Design review of the part built by this model. Coordinates are the model's own, in mm. A direction names the side the tool comes from. Round coordinates to 2 decimals unless told otherwise and drop trailing zeros. Write each loop counter-clockwise with the first axis right and the second up, starting at its lowest first coordinate (ties: lowest second). Pieces come first, ordered by that corner, then holes. Notation, with made-up numbers: (81, -5) -> (101, -5) arc R24 cw to (101, 26) -> close; hole circle Ø1 at (52, -14). An arc over 180 degrees is marked (long way). Write item = value, one per line. Start each with the question number.
Item 1: Add section D-D, the plane x = 132. State the section outline as (y, z) points.
Item 2: Add section C-C, the plane z = 96. State the section outline as (x, y) points, then the cut area to 3 significant figures.
Item 3: Add section B-B, the plane x = 15. State the section outline as (y, z) points (3 decimals).
Item 4: Add section A-A, the plane y = -4.25. State how many separate pieces and enclosed holes the cut face has, then the cut area to 3 significant figures.
Item 5: To check wall thickness, follow L1, parallel to X at y = -1.5, z = -26.5 (3 decimals); L2, parallel to X at y = -2.5, z = 23 (3 decimals); L3, parallel to Z at x = 15, y = -5.1 (3 decimals). State the ranges of each line that lie inside material, in increasing order.
Item 6: For pin 1 Ø10 at (x, z) = (-15, 25.98) entering from +Y; pin 2 Ø4 at (x, z) = (15, -25.98) entering from +Y; pin 3 Ø8.5 at (x, z) = (-30, 0) entering from +Y, all flat-tipped, find the tip position at first contact; note any pin that passes through.
Item 7: Mouldability with a two-part tool opening along X and no side actions: class faces 3 (the flat face through (-60, -3, 169.625)), 4 (the conical face through (-18.27, -2.95, 26.71)), 5 (the cylindrical face through (-71.484, -3.131, -69.929)) as released by +X, released by -X, zero draft, split by the parting line, or undercut.
Item 8: Machinability: for faces 1 (the flat face through (-20, -3, 123)), 2 (the conical face through (33.32, -2.95, 0.44)), which of the approach directions +Z, -Z, +X, -X, +Y, -Y give a long, thin tool a straight path to every point of the face, cutting with its end or side? Answer none if there is none.
from build123d import *

# Parameters (mm, degrees)
BOSS_EXTRUDE1_DEPTH                             = 6.35
FILLET1_R                                       = 5
TAP_DRILL_FOR_M6X1_0_TAP1_D                     = 5
CSK_FOR_M6_FLAT_HEAD_MACHINE_SCREW1_D           = 6.4
CSK_FOR_M6_FLAT_HEAD_MACHINE_SCREW1_CSINK_D     = 12.6
CSK_FOR_M6_FLAT_HEAD_MACHINE_SCREW1_CSINK_ANGLE = 90


with BuildPart() as part:
    # Sketch1 → Boss-Extrude1 (new body)
    with BuildSketch(Plane(origin=(0, 0, 0), x_dir=(1, 0, 0), z_dir=(0, 1, 0))):
        with BuildLine():
            Line((0, 100), (169.625, 100))
            Line((169.625, 100), (169.625, 20))
            Line((169.625, 20), (79.625, 20))
            Line((79.625, 20), (-20, -79.625))
            Line((-20, -79.625), (-20, -169.625))
            Line((-20, -169.625), (-100, -169.625))
            Line((-100, -169.625), (-100, 0))
            ThreePointArc((-100, 0), (-70.710678119, 70.710678119), (0, 100))
        make_face()
    extrude(amount=-BOSS_EXTRUDE1_DEPTH)

    # Fillet1
    fillet1_edges = [part.edges().sort_by_distance(p)[0] for p in [
        (169.625, -3.175, -20),
        (79.625, -3.175, -20),
        (-20, -3.175, 79.625),
        (-20, -3.175, 169.625),
        (-100, -3.175, 169.625),
        (169.625, -3.175, -100),
    ]]
    fillet(fillet1_edges, radius=FILLET1_R)

    # Tap Drill for M6x1.0 Tap1 (through all)
    with Locations(Plane(origin=(82.8, 0, -90), x_dir=(0, 0, 1), z_dir=(0, 1, 0))):
        with Locations((0, 0), (0, 70), (60, 70), (172.8, -172.8), (172.8, -112.8), (242.8, -112.8), (242.8, -172.8), (60, 0)):
            Hole(TAP_DRILL_FOR_M6X1_0_TAP1_D / 2)

    # CSK for M6 Flat Head Machine Screw1 (through all)
    with Locations(Plane(origin=(15, 0, -25.980762114), x_dir=(0, 0, 1), z_dir=(0, 1, 0))):
        with Locations((0, 0), (25.980762114, 15), (51.961524228, 0), (51.961524228, -30), (25.980762114, -45), (0, -30)):
            CounterSinkHole(CSK_FOR_M6_FLAT_HEAD_MACHINE_SCREW1_D / 2, CSK_FOR_M6_FLAT_HEAD_MACHINE_SCREW1_CSINK_D / 2, counter_sink_angle=CSK_FOR_M6_FLAT_HEAD_MACHINE_SCREW1_CSINK_ANGLE)


solid = part.part
Result set:
q1.outline = (-6.35, -100) -> (0, -100) -> (0, -20) -> (-6.35, -20) -> close
q2.outline = (-100, -6.35) -> (-20, -6.35) -> (-20, 0) -> (-100, 0) -> close
q2.area = 508 mm²
q3.outline = (-6.35, -100) -> (0, -100) -> (0, -32.281) -> (-3.1, -29.181) -> (-6.35, -29.181) -> close; (-6.35, -22.781) -> (-3.1, -22.781) -> (0, -19.681) -> (0, 19.681) -> (-3.1, 22.781) -> (-6.35, 22.781) -> close; (-6.35, 29.181) -> (-3.1, 29.181) -> (0, 32.281) -> (0, 44.625) -> (-6.35, 44.625) -> close
q4.separate_pieces = 1
q4.enclosed_holes = 14
q4.area = 39,200 mm²
q5.L1 = -96.425 to -19.772, -10.228 to 10.228, 19.772 to 169.625
q5.L2 = -100 to -17.357, -12.643 to 12.643, 17.357 to 36.625
q5.L3 = -100 to -29.181, -22.781 to 22.781, 29.181 to 44.625
q6.pin_1 = -1.3
q6.pin_2 = through
q6.pin_3 = -2.05
q7.face_3 = zero draft
q7.face_4 = undercut
q7.face_5 = released by -X
q8.face_1 = +Z, +X, +Y, -Y
q8.face_2 = +Y
